from build123d import *

# Parameters (mm, degrees)
F0_W     = 23.84
F0_H     = 1.58
F1_DEPTH = 7
F2_R     = 1.5
F3_DEPTH = 25
F4_R     = 1.5
F5_DEPTH = 25


with BuildPart() as f1:
    # F0 (on Top) → F1 (new body)
    with BuildSketch(Plane.XY):
        Polygon((0, 25.42), (0, 0), (1.58, 0), (1.58, 1.58), (1.58, 25.42), align=None)
        with Locations((13.5, 0.79)):
            Rectangle(F0_W, F0_H)
    extrude(amount=F1_DEPTH)

    # F2 (on face) → F3 (cut)
    with BuildSketch(Plane(origin=(0, 0, 0), x_dir=(0, -1, 0), z_dir=(-1, 0, 0))):
        with Locations((-20, 3.5)):
            Circle(F2_R)
    extrude(amount=-F3_DEPTH, mode=Mode.SUBTRACT)

    # F4 (on face) → F5 (cut)
    with BuildSketch(Plane.XZ):
        with Locations((20, 3.5)):
            Circle(F4_R)
    extrude(amount=-F5_DEPTH, mode=Mode.SUBTRACT)


solid = f1.part
The listing builds one solid part. Answer for the finished solid, in the listing's coordinates (mm). A direction names the side the tool comes from. Round coordinates to 2 decimals unless told otherwise and drop trailing zeros. Order: outer loops, then holes, each group sorted by start corner. A loop starts at its lowest first (then second) coordinate and runs counter-clockwise, first axis right, second up. Notation, with made-up numbers: (54, 68.25) -> (108, 68.25) arc R15 cw to (108, 85.25) -> close; hole circle Ø1 at (50.25, -20.75). An arc over 180 degrees is marked (long way). Put each result on its own line as item: value.
Q1. Section D-D, the plane z = 5.75 is taken. Write down the section's boundary in (x, y), and give its area (3 significant figures).
Results list:
outline: (0, 0) -> (25.42, 0) -> (25.42, 1.58) -> (1.58, 1.58) -> (1.58, 25.42) -> (0, 25.42) -> close
area: 77.8 mm^2
Q2. Consider line 1 along Z through (x, y) = (0.75, 20); line 2 along X through (y, z) = (5.75, 2.75). Determine where each line is inside the solid, lowest interval first.
Results list:
line 1: 0 to 2, 5 to 7
line 2: 0 to 1.58
Q3. Each of these flat-tipped pins is pushed along its axis until it touches: P1, Ø3, axis at y = 17, z = 3, coming from the -X side; P2, Ø3.5, axis at y = 12.5, z = 4.5, coming from the +X side. Where does it stop, or does it pass through?
Results list:
P1: x = 0
P2: x = 1.58
Q4. Section C-C, the plane z = 2.5 is taken. Write down the section's boundary in (x, y).
Results list:
outline: (0, 0) -> (18.88, 0) -> (18.88, 1.58) -> (1.58, 1.58) -> (1.58, 18.88) -> (0, 18.88) -> close; (0, 21.12) -> (1.58, 21.12) -> (1.58, 25.42) -> (0, 25.42) -> close; (21.12, 0) -> (25.42, 0) -> (25.42, 1.58) -> (21.12, 1.58) -> close
Q5. Which of the six approach directions +Z, -Z, +X, -X, +Y, -Y give full straight-line access (tool end or side, diameter ignored) to faces 4 (the flat face through (1.58, 13, 3)), 5 (the flat face through (1, 7, 0))?
Results list:
face 4: +Z, -Z, +X, +Y
face 5: -Z, +X, -X, +Y, -Y
Q6. Determine the mould class of faces 1 (the flat face through (13, 0, 3)), 2 (the cylindrical face through (0.78, 21.5, 3.57)), 3 (the flat face through (1, 7, 7)) for opening direction Z: pulls with the +Z half, pulls with the -Z half, needs draft (parallel to the pull), parting line crosses it, or undercut.
Results list:
face 1: needs draft
face 2: undercut
face 3: pulls with the +Z half
Q7. Section A-A, the plane x = 20 is taken. Write down the section's boundary in (y, z), and give its area (3 significant figures).
Results list:
outline: (0, 0) -> (1.58, 0) -> (1.58, 2) -> (0, 2) -> close; (0, 5) -> (1.58, 5) -> (1.58, 7) -> (0, 7) -> close
area: 6.32 mm^2
